Source: three-view drawing plus pictorial views. Frame: mm from the lowest corner of the part. A direction names the side the tool comes from. Round coordinates to 2 decimals unless told otherwise and drop trailing zeros. Loops run counter-clockwise (first coordinate to the right, second up) from the corner with the lowest first, then second, coordinate; pieces in that order, holes last. Notation, with made-up numbers: (37, 38.5) -> (50, 38.5) arc R25 cw to (50, 59.5) -> close; hole circle Ø11 at (37.5, 20). An arc over 180 degrees is marked (long way). Answer as a JSON object with one key per item and string values. Group by question number.
Item 1: Section query C-C on y = 23. Return loops of the section in (x, z), and give its area (3 significant figures).
Item 2: Set-up query: the marked faces 1, 2, 3 and 4. Return all of +Z, -Z, +X, -X, +Y, -Y with unobstructed straight access to the full face (end or side cutting, diameter ignored); none if empty.
Item 3: Draft query along Y for the marked faces 5, 6, 7 and 8. Return one class per face: released by +Y, released by -Y, zero draft, split by the parting line, or undercut.
Item 4: Section query A-A on z = 11.5. Return loops of the section in (x, y).
Item 5: Section query B-B on z = 54.5. Return loops of the section in (x, y), and give its area (3 significant figures).
Item 6: Pin query (flat end, axial travel): pin 1 (7.5 mm diameter, centred on x = 92, z = 35.5, fed in from -Y); pin 2 (12.5 mm diameter, centred on x = 88, z = 31, fed in from +Y); pin 3 (3 mm diameter, centred on y = 61.5, z = 14, fed in from +X). Return the tip coordinate at first contact, or that it passes through.
Item 7: Section query D-D on x = 24. Return loops of the section in (y, z).
Item 8: Material intervals for line 1 (Y direction, x = 49.5, z = 8); line 2 (X direction, y = 64, z = 7.5); line 3 (Z direction, x = 27, y = 81), sorted ascending. Write a range as [from, to].
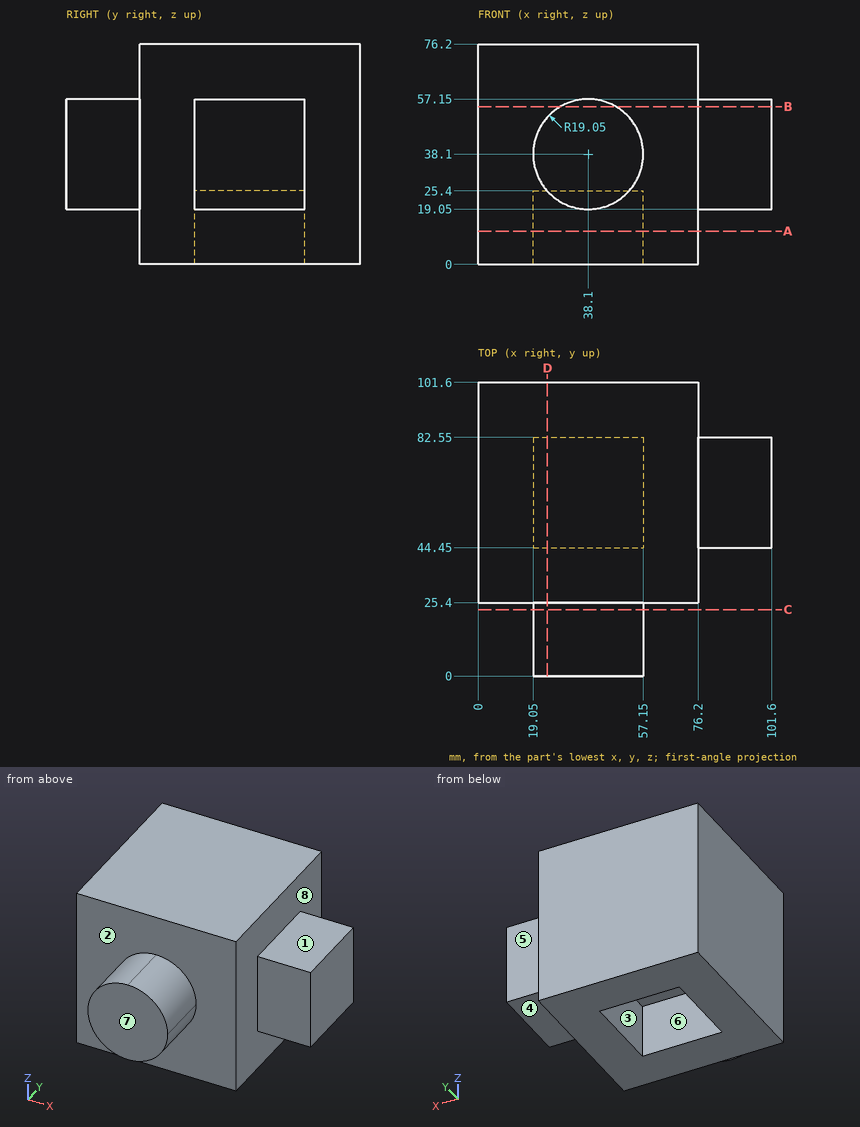
Solved:
{
 "1": {"outline": "(19.05, 38.1) arc R19.05 ccw (long way) to (38.1, 57.15) arc R19.05 ccw to start", "area": "1,140 mm²"},
 "2": {"face 1": "+Z, +X, +Y, -Y", "face 2": "-Y", "face 3": "-Z", "face 4": "-Z, +X, +Y, -Y"},
 "3": {"face 5": "released by +Y", "face 6": "undercut", "face 7": "released by -Y", "face 8": "zero draft"},
 "4": {"outline": "(0, 25.4) -> (76.2, 25.4) -> (76.2, 101.6) -> (0, 101.6) -> close; hole (19.05, 44.45) -> (57.15, 44.45) -> (57.15, 82.55) -> (19.05, 82.55) -> close"},
 "5": {"outline": "(0, 25.4) -> (28.41, 25.4) -> (28.41, 0) -> (47.79, 0) -> (47.79, 25.4) -> (76.2, 25.4) -> (76.2, 44.45) -> (101.6, 44.45) -> (101.6, 82.55) -> (76.2, 82.55) -> (76.2, 101.6) -> (0, 101.6) -> close", "area": "7,270 mm²"},
 "6": {"pin 1": "y = 44.45", "pin 2": "y = 82.55", "pin 3": "x = 76.2"},
 "7": {"outline": "(0, 25.29) -> (25.4, 25.29) -> (25.4, 0) -> (44.45, 0) -> (44.45, 25.4) -> (82.55, 25.4) -> (82.55, 0) -> (101.6, 0) -> (101.6, 76.2) -> (25.4, 76.2) -> (25.4, 50.91) -> (0, 50.91) -> close"},
 "8": {"line 1": "[25.4, 44.45], [82.55, 101.6]", "line 2": "[0, 19.05], [57.15, 76.2]", "line 3": "[25.4, 76.2]"}
}
